```python
from build123d import *

# Parameters (mm, degrees)
BOSS_EXTRUDE1_DEPTH = 4
SKETCH3_R           = 1.5
BOSS_EXTRUDE3_DEPTH = 4
LPATTERN2_COUNT     = 2
LPATTERN2_PITCH     = 38
FILLET1_DEPTH       = 4


with BuildPart() as part:
    # Sketch1 → Boss-Extrude1 (new body)
    with BuildSketch(Plane.XY):
        Polygon((23.699409247, -33.383107264), (23.015368961, -31.503722023), (70, -14.402714856), (70, -16.531070401), align=None)
        Polygon((68, -15.130655325), (70, -14.402714856), (70, 28.358983849), (68, 29.513684387), align=None)
    extrude(amount=BOSS_EXTRUDE1_DEPTH)

    # Sketch3 → Boss-Extrude3 (add)
    # profile 1 of 3: a face of its own
    with BuildSketch(Plane(origin=(0, 0, 0), x_dir=(-1, 0, 0), z_dir=(0, 0, -1))):
        with BuildLine():
            ThreePointArc((-33.133334302, -32.988363728), (-31.041480631, -37.474358403), (-26.555485957, -35.382504732))
            ThreePointArc((-26.555485957, -35.382504732), (-26.397582994, -34.793202852), (-26.34441013, -34.18543423))
            ThreePointArc((-26.34441013, -34.18543423), (-26.503443688, -33.142389054), (-26.96609198, -32.194131985))
            Line((-26.96609198, -32.194131985), (-30.769345343, -30.809860967))
            ThreePointArc((-30.769345343, -30.809860967), (-32.216249353, -31.61164739), (-33.133334302, -32.988363728))
        make_face()
        with Locations((-29.84441013, -34.18543423)):
            Circle(SKETCH3_R, mode=Mode.SUBTRACT)
    # profile 2 of 3: a face of its own
    with BuildSketch(Plane(origin=(0, 0, 0), x_dir=(-1, 0, 0), z_dir=(0, 0, -1))):
        with BuildLine():
            ThreePointArc((-26.34441013, -34.18543423), (-26.397582994, -34.793202852), (-26.555485957, -35.382504732))
            Line((-26.555485957, -35.382504732), (-25.578794489, -32.699066978))
            Line((-25.578794489, -32.699066978), (-26.96609198, -32.194131985))
            ThreePointArc((-26.96609198, -32.194131985), (-26.503443688, -33.142389054), (-26.34441013, -34.18543423))
        make_face()
    # profile 3 of 3: a face of its own
    with BuildSketch(Plane(origin=(0, 0, 0), x_dir=(-1, 0, 0), z_dir=(0, 0, -1))):
        with BuildLine():
            Line((-32.156642834, -30.304925974), (-33.133334302, -32.988363728))
            ThreePointArc((-33.133334302, -32.988363728), (-32.216249353, -31.61164739), (-30.769345343, -30.809860967))
            Line((-30.769345343, -30.809860967), (-32.156642834, -30.304925974))
        make_face()
    boss_extrude3 = extrude(amount=-BOSS_EXTRUDE3_DEPTH)

    # LPattern2: Boss-Extrude3 ×2
    with Locations(*[Vector(0.9396926207859079, 0.3420201433256704, 0) * (i * LPATTERN2_PITCH) for i in range(1, LPATTERN2_COUNT)]):
        add(boss_extrude3)

    # Fillet1: read off the stored shape, not the designer's step
    # Fillet1 outline → Fillet1 (add)
    with BuildSketch(Plane.XY):
        with BuildLine():
            ThreePointArc((68.841653892, -19.991598282), (68.990249602, -20.53029423), (69.051216895, -21.085773301))
            ThreePointArc((69.051216895, -21.085773301), (69.257041708, -18.75247713), (70, -16.531070401))
            Line((70, -16.531070401), (67.864962424, -17.308160528))
            Line((67.864962424, -17.308160528), (68.841653892, -19.991598282))
        make_face()
        with BuildLine():
            Line((61.287114079, -19.702301531), (53.812215852, -22.42294199))
            ThreePointArc((53.812215852, -22.42294199), (58.800886589, -21.943638956), (63.395611681, -23.944905669))
            ThreePointArc((63.395611681, -23.944905669), (62.720311337, -23.244734469), (62.263805547, -22.385739285))
            Line((62.263805547, -22.385739285), (61.287114079, -19.702301531))
        make_face()
        with BuildLine():
            ThreePointArc((33.133334302, -32.988363728), (33.33578204, -33.939828481), (33.268533335, -34.910265432))
            ThreePointArc((33.268533335, -34.910265432), (35.501907513, -30.423773828), (39.631541062, -27.584285515))
            Line((39.631541062, -27.584285515), (32.156642834, -30.304925974))
            Line((32.156642834, -30.304925974), (33.133334302, -32.988363728))
        make_face()
        with BuildLine():
            ThreePointArc((23.699409247, -33.383107264), (25.524081147, -34.637762706), (27.027892588, -36.263228478))
            ThreePointArc((27.027892588, -36.263228478), (26.760091208, -35.839815319), (26.555485957, -35.382504732))
            Line((26.555485957, -35.382504732), (25.578794489, -32.699066978))
            Line((25.578794489, -32.699066978), (23.699409247, -33.383107264))
        make_face()
    extrude(amount=FILLET1_DEPTH)


solid = part.part
```
Could you check a few things on this model? Use its own coordinates, in mm. A direction names the side the tool comes from. Round coordinates to 2 decimals unless told otherwise and drop trailing zeros. Order: outer loops, then holes, each group sorted by start corner. A loop starts at its lowest first (then second) coordinate and runs counter-clockwise, first axis right, second up. Notation, with made-up numbers: M 39.25,54 L 85.25,54 A17 ccw 85.25,71 Z; hole C 1.5,86 d10. An arc over 180 degrees is marked long. One line per question, with ' | ' between items. Start each with the question number.
(1) For faces 1 (the face through (46.82, -24.97, 1.97)), 2 (the face through (25.501, -34.617, 1.972)), 3 (the face through (68, 8, 2)), which set-ups out of +Z, -Z, +X, -X, +Y, -Y let a thin tool reach every point of the face, with its end or its side?
(2) Thinking about a two-plate mould opening in X: for faces 4 (the face through (64.12, -20.74, 1.97)), 5 (the face through (69.25, -18.78, 1.97)), 6 (the face through (28.414, -33.735, 1.972)), 7 (the face through (23.362, -32.457, 1.972)), which applies, +X half, -X half, draft (parallel to the pull), parting line (faces both ways), or undercut?
(3) Suppose I cut it at C-C on x = 35. List the corners of the cut face in (y, z) for me, then the cut area to 3 significant figures.
(4) Suppose I cut it at A-A on z = 1.75. List the corners of the cut face in (x, y) for me, then the cut area to 3 significant figures.
(5) Please list where these lines run through material, in increasing order: line 1 along X through (y, z) = (20.5, 3.1); line 2 along Y through (x, z) = (56, 1.25); line 3 along Y through (x, z) = (46, 3.15).
(6) For P1, Ø1, axis at y = -5, z = 2, coming from the -X side; P2, Ø1.5, axis at x = 41, z = 2.5, coming from the -Y side, each with a flat end and sliding along its axis, tell me the tip position at first contact or that it passes through.
(7) Suppose I cut it at B-B on y = -7.5. List the corners of the cut face in (x, z) for me.
Geometry results:
1) face 1: +Z, -Z, -Y | face 2: +Z, -Z, -X, -Y | face 3: +Z, -Z, -X, +Y
2) face 4: undercut | face 5: +X half | face 6: undercut | face 7: -X half
3) outline: M -31.05,0 L -27.14,0 L -27.14,4 L -31.05,4 Z | area: 15.6 mm²
4) outline: M 23.02,-31.5 L 23.7,-33.38 A10 cw 27.03,-36.26 A3.5 ccw 33.27,-34.91 A10 cw 39.63,-27.58 L 53.81,-22.42 A10 cw 63.4,-23.94 A3.5 ccw 69.05,-21.09 A10 cw 70,-16.53 L 70,28.36 L 68,29.51 L 68,-15.13 Z; hole C 29.84,-34.19 d3; hole C 65.55,-21.19 d3 | area: 276 mm²
5) line 1: 68 to 70 | line 2: -21.9 to -19.5 | line 3: -25.27 to -23.14
6) P1: x = 68 | P2: y = -27.36
7) outline: M 68,0 L 70,0 L 70,4 L 68,4 Z
